For this review, take the finished solid that the model builds, in its own axes (mm). A direction names the side the tool comes from. Round coordinates to 2 decimals unless told otherwise and drop trailing zeros. Write each loop counter-clockwise with the first axis right and the second up, starting at its lowest first coordinate (ties: lowest second). Pieces come first, ordered by that corner, then holes. Notation, with made-up numbers: (0.25, 7.5) -> (50.25, 7.5) arc R12 cw to (50.25, 15.5) -> close; hole circle Ø11 at (25.5, 22). An arc over 180 degrees is marked (long way). Write each question's results on one line, items separated by ' | '. Start each with the question number.
Item 1: Add section B-B (y = -12.18). State the section outline as (x, z) points (3 decimals).
Item 2: Add section D-D (x = 26). State the section outline as (y, z) points.
Item 3: Add section C-C (z = 101.25). State the section outline as (x, y) points (3 decimals).
Item 4: Clearance check with flat-ended pins moving along their axes: pin 1 (2.5 mm diameter, centred on x = -25.555, y = -12.18, fed in from +Z); pin 2 (12 mm diameter, centred on x = -22, y = -22, fed in from +Z); pin 3 (0.8 mm diameter, centred on x = -7.5, y = -71, fed in from +Z); pin 4 (1.5 mm diameter, centred on x = 19, z = 47.5, fed in from -Y). State where each tip first meets the part, or that it passes through.
Item 5: Add section A-A (z = 7). State the section outline as (x, y) points, plus the area to 3 significant figures.
Item 6: Tool access review of faces 4 (the flat face through (0, -35, 1.5)), 5 (the cylindrical face through (-25.08, -0.74, 99.34)), 6 (the cylindrical face through (-25.25, -0.74, 16.09)), 7 (the flat face through (11, -80.5, 7)), 8 (the cylindrical face through (-8.265, -75.937, 7.94)): name each direction out of +Z, -Z, +X, -X, +Y, -Y from which nothing blocks a thin tool from reaching the whole face with its end or side.
Item 7: To check wall thickness, follow line 1 along Z through (x, y) = (-25.5, -0.65) (3 decimals); line 2 along Z through (x, y) = (-21, -59); line 3 along Y through (x, z) = (12.5, 63). State the ranges of each line that lie inside material, in increasing order.
Item 8: The part is to be moulded in two halves that separate along X. For faces 1 (the flat face through (-31.83, -1, 52)), 2 (the cylindrical face through (14.235, -75.937, 7.94)), 3 (the flat face through (-11, -80.5, 7)), say which applies: +X half, -X half, draft (parallel to the pull), parting line (faces both ways), or undercut.
from build123d import *

# Parameters (mm, degrees)
F1_DEPTH      = 31.83
F1_DEPTH_BACK = 31.83
F2_R          = 1.955
F3_DEPTH      = 25
F4_R          = 3.13
F5_DEPTH      = 9
F6_R          = 1.95
F7_DEPTH      = 25


with BuildPart() as f1:
    # F0 (on Right) → F1 (new body, two sides)
    with BuildSketch(Plane.YZ) as f1_sk:
        Polygon((0, 0), (0, 111.5), (-1.5, 111.5), (-1.5, 1.5), (-70, 1.5), (-70, 14), (-71.5, 14), (-71.5, 0), align=None)
    extrude(amount=F1_DEPTH)
    extrude(f1_sk.sketch, amount=-F1_DEPTH_BACK)

    # F2 (on face) → F3 (cut)
    with BuildSketch(Plane(origin=(0, 0, 0), x_dir=(-1, 0, 0), z_dir=(0, 1, 0))):
        with Locations((-25.5, 101.25)):
            Circle(F2_R)
        with Locations((25.5, 101.25)):
            Circle(F2_R)
        with Locations((25.5, 14.15)):
            Circle(F2_R)
        with Locations((-25.5, 14.15)):
            Circle(F2_R)
    extrude(amount=-F3_DEPTH, mode=Mode.SUBTRACT)

    # F4 (on face) → F5 (join)
    with BuildSketch(Plane.XZ.offset(71.5)):
        with Locations((-11.25, 7)):
            Circle(F4_R)
        with Locations((11.25, 7)):
            Circle(F4_R)
    extrude(amount=F5_DEPTH)

    # F6 (on face) → F7 (cut)
    with BuildSketch(Plane(origin=(0, 0, 0), x_dir=(1, 0, 0), z_dir=(0, 0, -1))):
        with Locations((-25.555, 44.25)):
            Circle(F6_R)
        with Locations((25.555, 44.25)):
            Circle(F6_R)
        with Locations((25.555, 12.18)):
            Circle(F6_R)
        with Locations((-25.555, 12.18)):
            Circle(F6_R)
    extrude(amount=-F7_DEPTH, mode=Mode.SUBTRACT)


solid = f1.part
Responses:
1) outline: (-31.83, 0) -> (-27.505, 0) -> (-27.505, 1.5) -> (-31.83, 1.5) -> close; (-23.605, 0) -> (23.605, 0) -> (23.605, 1.5) -> (-23.605, 1.5) -> close; (27.505, 0) -> (31.83, 0) -> (31.83, 1.5) -> (27.505, 1.5) -> close
2) outline: (-71.5, 0) -> (-46.15, 0) -> (-46.15, 1.5) -> (-70, 1.5) -> (-70, 14) -> (-71.5, 14) -> close; (-42.35, 0) -> (-14.08, 0) -> (-14.08, 1.5) -> (-42.35, 1.5) -> close; (-10.28, 0) -> (0, 0) -> (0, 12.26) -> (-1.5, 12.26) -> (-1.5, 1.5) -> (-10.28, 1.5) -> close; (-1.5, 16.04) -> (0, 16.04) -> (0, 99.36) -> (-1.5, 99.36) -> close; (-1.5, 103.14) -> (0, 103.14) -> (0, 111.5) -> (-1.5, 111.5) -> close
3) outline: (-31.83, -1.5) -> (-27.455, -1.5) -> (-27.455, 0) -> (-31.83, 0) -> close; (-23.545, -1.5) -> (23.545, -1.5) -> (23.545, 0) -> (-23.545, 0) -> close; (27.455, -1.5) -> (31.83, -1.5) -> (31.83, 0) -> (27.455, 0) -> close
4) pin 1: passes through | pin 2: stops at z = 1.5 | pin 3: stops at z = 14 | pin 4: stops at y = -1.5
5) outline: (-31.83, -71.5) -> (-14.38, -71.5) -> (-14.38, -80.5) -> (-8.12, -80.5) -> (-8.12, -71.5) -> (8.12, -71.5) -> (8.12, -80.5) -> (14.38, -80.5) -> (14.38, -71.5) -> (31.83, -71.5) -> (31.83, -70) -> (-31.83, -70) -> close; (-31.83, -1.5) -> (31.83, -1.5) -> (31.83, 0) -> (-31.83, 0) -> close | area: 304 mm^2
6) face 4: +Z, +X, -X | face 5: +Y, -Y | face 6: +Y | face 7: +Z, -Z, +X, -X, -Y | face 8: -Y
7) line 1: z = 0 to 12.195, 16.105 to 99.295, 103.205 to 111.5 | line 2: z = 0 to 1.5 | line 3: y = -1.5 to 0
8) face 1: -X half | face 2: undercut | face 3: draft
